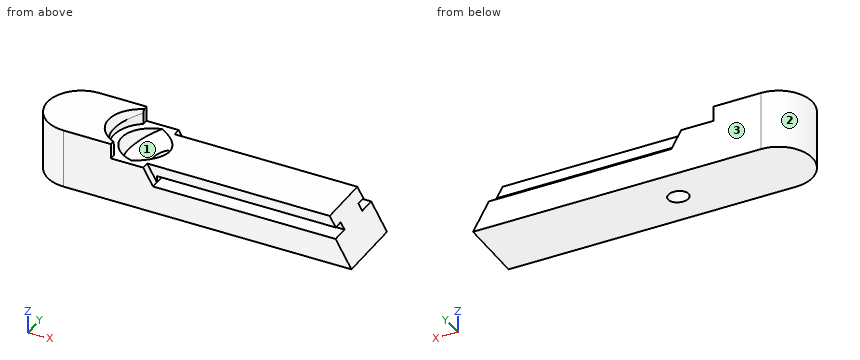
```python
from build123d import *

# Parameters (mm, degrees)
F1_DEPTH  = 5.969
F3_DEPTH  = 1.016
F4_W      = 26.6201772846
F4_H      = 0.889
F5_DEPTH  = 1.27
F7_DEPTH  = 9.145
F10_DEPTH = 2.032


with BuildPart() as f1:
    # F0 (on Top) → F1 (new body)
    with BuildSketch(Plane.XY):
        with BuildLine():
            Line((25.1714, 4.572), (-13.4366, 4.572))
            ThreePointArc((-13.4366, 4.572), (-18.0086, 0), (-13.4366, -4.572))
            Line((-13.4366, -4.572), (25.1714, -4.572))
            Line((25.1714, -4.572), (25.1714, 4.572))
        make_face()
    extrude(amount=F1_DEPTH)

    # F2 (on face) → F3 (cut)
    with BuildSketch(Plane.XZ.offset(4.572)):
        Polygon((-2.7686, 5.969), (-1.4487772846, 3.683), (25.1714, 3.683), (25.1714, 5.969), align=None)
    extrude(amount=-F3_DEPTH, mode=Mode.SUBTRACT)

    # F4 (on face) → F5 (cut)
    with BuildSketch(Plane.XZ.offset(3.556)):
        with Locations((11.8613113577, 4.1275)):
            Rectangle(F4_W, F4_H)
    extrude(amount=-F5_DEPTH, mode=Mode.SUBTRACT)

    # F6 (on face) → F7 (cut, through all)
    with BuildSketch(Plane.XZ.offset(4.572)):
        Polygon((21.7251962432, 5.969), (25.1714, 0), (25.1714, 5.969), align=None)
    extrude(amount=-F7_DEPTH, mode=Mode.SUBTRACT)

    # F8: F1 across plane


with BuildPart() as f1_1:
    add(f1.part)
    add(f1.part.mirror(Plane.XZ), mode=Mode.INTERSECT)

    # F9 (on face) → F10 (join)
    with BuildSketch(Plane.XY.offset(5.969)):
        with BuildLine():
            Line((-7.0992680903, 4.572), (-13.4366, 4.572))
            ThreePointArc((-13.4366, 4.572), (-18.0086, 0), (-13.4366, -4.572))
            Line((-13.4366, -4.572), (-7.0992680903, -4.572))
            Line((-7.0992680903, -4.572), (-7.0992680903, -3.81))
            ThreePointArc((-7.0992680903, -3.81), (-9.144, 0), (-7.0992680903, 3.81))
            Line((-7.0992680903, 3.81), (-7.0992680903, 4.572))
        make_face()
    extrude(amount=F10_DEPTH)

    # F11 (on Front) → F12 (revolve, cut)
    with BuildSketch(Plane.XZ):
        Polygon((1.905, -3.2995567884), (0, 0), (-7.366, 12.7582862486), (-11.2594770103, 10.5103862486), (-8.6375064372, 5.969), (-8.0509185637, 5.969), (-7.1927008583, 4.4825233303), (-3.8830387258, 4.3380203608), (0.871138873, -3.8964567884), align=None)
    revolve(axis=Axis((-3.683, 0, 6.3791431243), (-0.5, 0, 0.8660254038)), mode=Mode.SUBTRACT)


solid = f1_1.part
```
Could you check a few things on this model? Use its own coordinates, in mm. Face numbers are marked on the shaded views. Give positions to 0.01 mm unless a question says otherwise; leave off trailing zeros. Loops run counter-clockwise (first coordinate to the right, second up) from the corner with the lowest first, then second, coordinate; pieces in that order, holes last. Notation, with made-up numbers: (2, -5) - (44, -5) arc R17 cw to (44, 0) - close; hole circle Ø9 at (-22, 18.5). An arc over 180 degrees is marked (long way). Answer in a Markdown table with one row per item. Add a question column.
Q1. Please list where these lines run through material, in increasing order: L1, parallel to Z at x = 11, y = -2.5; L2, parallel to Z at x = 13, y = 0.75; L3, parallel to Y at x = 4.5, z = 5. Write a range as from..to.
Q2. We'd pull the mould along X, two halves only. Please class the marked faces 1, 2 and 3: +X half, -X half, draft (parallel to the pull), parting line (faces both ways), or undercut.
Q3. If we section it at A-A (y = 0): List the corners of the cut face in (x, z) for me, plus the area to 3 significant figures.
Q4. For pin 1 (1.8 mm diameter, centred on x = 15.5, y = 3, fed in from +Z); pin 2 (1 mm diameter, centred on y = -2.5, z = 6, fed in from +X); pin 3 (0.6 mm diameter, centred on y = -4, z = 6.5, fed in from +X), each with a flat end and sliding along its axis, tell me the tip position at first contact or that it passes through.
Q5. If we section it at B-B (x = 5): List the corners of the cut face in (y, z) for me, plus the area to 3 significant figures.
The answers:
| question | item | result |
|---|---|---|
| 1 | L1 | z = 0..3.68, 4.57..5.97 |
| 1 | L2 | z = 0..5.97 |
| 1 | L3 | y = -3.56..3.56 |
| 2 | face 1 | undercut |
| 2 | face 2 | -X half |
| 2 | face 3 | draft |
| 3 | outline | (-18.01, 0) - (-1.38, 0) - (-3.88, 4.34) - (-7.19, 4.48) - (-8.05, 5.97) - (-9.14, 5.97) - (-9.14, 6.85) - (-9.81, 8) - (-18.01, 8) - close; (-1.82, 5.53) - (1.38, 0) - (25.17, 0) - (21.73, 5.97) - (-1.59, 5.97) - close |
| 3 | area | 243 mm^2 |
| 4 | pin 1 | stops at z = 5.97 |
| 4 | pin 2 | stops at x = 22 |
| 4 | pin 3 | stops at x = -7.1 |
| 5 | outline | (-4.57, 0) - (4.57, 0) - (4.57, 3.68) - (2.29, 3.68) - (2.29, 4.57) - (3.56, 4.57) - (3.56, 5.97) - (-3.56, 5.97) - (-3.56, 4.57) - (-2.29, 4.57) - (-2.29, 3.68) - (-4.57, 3.68) - close |
| 5 | area | 47.7 mm^2 |
